For this review, take the finished solid that the model builds, in its own axes (mm). Face numbers are marked on the shaded views. A direction names the side the tool comes from. Round coordinates to 2 decimals unless told otherwise and drop trailing zeros. Order: outer loops, then holes, each group sorted by start corner. A loop starts at its lowest first (then second) coordinate and runs counter-clockwise, first axis right, second up. Notation, with made-up numbers: M 20,50 L 37,50 A14 cw 37,59 Z; hole C 56.25,-30.75 d1. An arc over 180 degrees is marked long. Put each result on its own line as item: value.
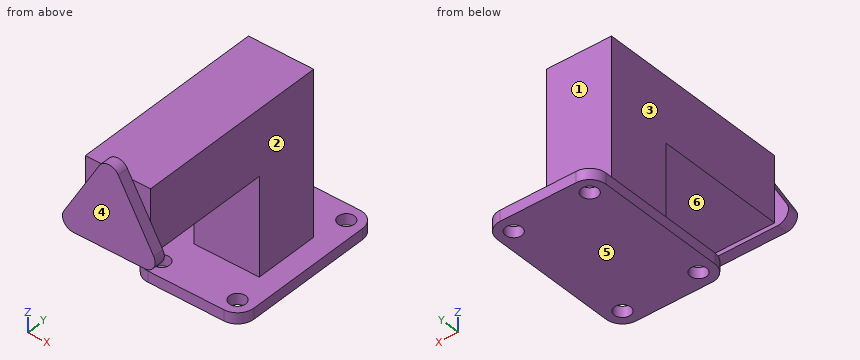
Autodesk Fusion 360 part; units mm, degrees
sketch "Sketch1" plane through (0, 0, 0) normal (0, 0, 1) x (1, 0, 0) in component "Mounting Plate1"
  line L0 (-50, 75) -> (50, 75)
  line L1 (50, 75) -> (50, -75)
  line L2 (50, -75) -> (-50, -75)
  line L3 (-50, -75) -> (-50, 75)
  line L4 (-50, 75) -> (50, -75) construction
  line L5 (50, 75) -> (-50, -75) construction
  circle A0 centre (-35, 60) radius 7.5
  circle A1 centre (35, 60) radius 7.5
  line L6 (0, 0) -> (21.7934, 0) construction
  circle A2 centre (-35, -60) radius 7.5
  circle A3 centre (35, -60) radius 7.5
  dimension "d1" = 100
  dimension "d2" = 150
  dimension "d3" = 15
  dimension "d4" = 15
  dimension "d5" = 15
  dimension "d6" = 15
extrude "Extrude1" add sketch "Sketch1" along normal blind 10 makes body 1 in component "Mounting Plate1"
fillet "Fillet1" radius 15 4 edges at (-50, 75, 5) (50, 75, 5) (50, -75, 5) (-50, -75, 5) on bodies 1 in component "Mounting Plate1"
ref_plane "WorkPlane1" through (0, -150, 0) normal (0, 1, 0) x (0, 0, 1) in component "Mounting Plate1"
sketch "Sketch2" plane through (0, -150, 0) normal (0, 1, 0) x (1, 0, 0) in component "Mounting Plate1"
  line L0 (-35, -10) -> (35, -10)
  line L1 (0, 0) -> (0, -125) construction
  line L2 (-50, -96.1325) -> (0, -182.735)
  line L3 (0, -182.735) -> (50, -96.1325)
  line L4 (50, -96.1325) -> (-50, -96.1325)
  point P0 (0, -125)
  dimension "d11" = 125
  dimension "d12" = 100
extrude "Extrude2" add sketch "Sketch2" against normal blind 10 separate body makes body 2 in component "Mounting Plate1"
fillet "Fillet2" radius 10 3 edges at (0, -155, 182.735) (50, -155, 96.1325) (-50, -155, 96.1325) on bodies 2 in component "Mounting Plate1"
sketch "Sketch1 (2)" plane through (0, 0, 10) normal (0, 0, 1) x (1, 0, 0)
  arc A0 (-50, -60) -> (-35, -75) centre (-35, -60) ccw
  line L0 (-35, -75) -> (35, -75)
  arc A1 (35, -75) -> (50, -60) centre (35, -60) ccw
  line L1 (50, -60) -> (50, 60)
  arc A2 (50, 60) -> (35, 75) centre (35, 60) ccw
  line L2 (35, 75) -> (-35, 75)
  arc A3 (-35, 75) -> (-50, 60) centre (-35, 60) ccw
  line L3 (-50, 60) -> (-50, -60)
  circle A4 centre (35, -60) radius 7.5
  circle A5 centre (-35, 60) radius 7.5
  circle A6 centre (-35, -60) radius 7.5
  circle A7 centre (35, 60) radius 7.5
  line L4 (-30, 30) -> (30, 30)
  line L5 (30, 30) -> (30, -30)
  line L6 (30, -30) -> (-30, -30)
  line L7 (-30, -30) -> (-30, 30)
  line L8 (-30, 30) -> (30, -30) construction
  line L9 (30, 30) -> (-30, -30) construction
extrude "Extrude3" add sketch "Sketch1 (2)" along normal blind 150 contours L4 L5 L6 L7 bodies 1 in component "Mounting Plate1"
sketch "Sketch2 (2)" plane through (0, -30, 0) normal (0, -1, 0) x (1, 0, 0)
  line L0 (-30, 10) -> (30, 10)
  line L1 (30, 10) -> (30, 160)
  line L2 (30, 160) -> (-30, 160)
  line L3 (-30, 160) -> (-30, 10)
  line L4 (-30, 160) -> (30, 160)
  line L5 (30, 160) -> (30, 100)
  line L6 (30, 100) -> (-30, 100)
  line L7 (-30, 100) -> (-30, 160)
extrude "Extrude4" add sketch "Sketch2 (2)" along normal blind 120 contours L1 L2 L3 L4 L5 L6 L7 bodies 1 2 in component "Mounting Plate1"
component "Mounting Plate1" placed x (1, 0, 0) y (0, 1, 0) z (0, 0, 1) at (0, 0, 0)
equation "d2 = ( 6 * 25 ) * 1 mm"
(1) Add section A-A on x = 0. Give the boundary of the cut face in (y, z) (1 decimal), then the cut area to 3 significant figures.
A:
outline: M -160,96.1 L -150,96.1 L -150,100 L -30,100 L -30,10 L -75,10 L -75,0 L 75,0 L 75,10 L 30,10 L 30,160 L -150,160 L -150,172.7 L -160,172.7 Z
area: 18,500 mm2
(2) Insertion check: pin 1 Ø3 at (y, z) = (30, 29) entering from -X; pin 2 Ø1 at (x, z) = (-23, 87.5) entering from -Y; pin 3 Ø8 at (x, y) = (1, 41.5) entering from +Z. Each pin has a flat end and moves straight along its axis. Give the tip position at first contact, or say it passes through.
A:
pin 1: stops at x = -30
pin 2: stops at y = -30
pin 3: stops at z = 10
(3) Draft analysis for pull direction Y (two halves, no side actions). For the marked faces 4, 5 and 6, state which applies: released by +Y, released by -Y, zero draft, split by the parting line, or undercut.
A:
face 4: released by -Y
face 5: zero draft
face 6: undercut
(4) To check wall thickness, follow L1, parallel to Y at x = 35, z = 8; L2, parallel to Z at x = -19, y = -62.5; L3, parallel to Z at x = 20, y = 66. State the ranges of each line that lie inside material, in increasing order.
A:
L1: y = -75 to -67.5, -52.5 to 52.5, 67.5 to 75
L2: z = 0 to 10, 100 to 160
L3: z = 0 to 10
(5) Add section D-D on z = 91. Give the boundary of the cut face in (x, y), then the cut area to 3 significant figures.
A:
outline: M -30,-30 L 30,-30 L 30,30 L -30,30 Z
area: 3,600 mm2
(6) For the marked faces 1, 2 and 3, list the 3-axis set-ups (+Z, -Z, +X, -X, +Y, -Y) from which the entire face can be reached by the end or side of a thin tool; tool diameter is ignored.
A:
face 1: +Z, +X, -X, +Y
face 2: +Z, +X, +Y
face 3: +Z, -X, +Y
(7) Add section C-C on z = 123. Give the boundary of the cut face in (x, y).
A:
outline: M -34.49,-160 L 34.49,-160 L 34.49,-150 L 30,-150 L 30,30 L -30,30 L -30,-150 L -34.49,-150 Z
(8) Add section B-B on y = -6.5. Give the boundary of the cut face in (x, z).
A:
outline: M -50,0 L 50,0 L 50,10 L 30,10 L 30,160 L -30,160 L -30,10 L -50,10 Z
